The model under review builds one solid part; all positions refer to its coordinate system, in mm. A direction names the side the tool comes from. Give positions to 0.01 mm unless a question says otherwise; leave off trailing zeros. Order: outer loops, then holes, each group sorted by start corner. A loop starts at its lowest first (then second) coordinate and runs counter-clockwise, first axis right, second up.
```python
from build123d import *

# Parameters (mm, degrees)
F0_R        = 18.7
F0_R_2      = 15.45
F1_DEPTH    = 20
F0_R_3      = 21
F2_DEPTH    = 5
F3_DEPTH    = 20
F4_S5_R     = 18.7
F4_T6_DEPTH = 31
F5_SIZE     = 3


# Not quite as in the source:
# - a fillet or chamfer that OpenCascade refuses, or shapes differently, is made with other operations: its cross-section is extruded or revolved along the edge and cut away or added


with BuildPart() as f1:
    # F0 (on Top) → F1 (new body)
    with BuildSketch(Plane.XY):
        Circle(F0_R)
        Circle(F0_R_2, mode=Mode.SUBTRACT)
    extrude(amount=F1_DEPTH)

    # F0 (on Top) → F2 (join)
    with BuildSketch(Plane.XY):
        Circle(F0_R_3)
        Circle(F0_R, mode=Mode.SUBTRACT)
    extrude(amount=F2_DEPTH)

    # F0 (on Top) → F3 (join)
    with BuildSketch(Plane.XY):
        Circle(F0_R_3)
        Circle(F0_R, mode=Mode.SUBTRACT)
    extrude(amount=-F3_DEPTH)

    # F4: chamfer of 2.5 on 1 edges, made by hand


with BuildPart() as f4_tool2:
    # F4_s3 → F4_t4 (revolve)
    with BuildSketch(Plane.XZ):
        Polygon((18.5, 5), (21, 2.5), (21, 5), align=None)
    revolve(axis=Axis((0, 0, 5), (0, 0, 1)))

    # F4_s5 → F4_t6 (cut, symmetric)
    with BuildSketch(Plane.XY.offset(3.8)):
        Circle(F4_S5_R)
    extrude(amount=F4_T6_DEPTH, both=True, mode=Mode.SUBTRACT)


with BuildPart() as f1_1:
    add(f1.part)

    # F4_t1: cut F4_tool2
    add(f4_tool2.part, mode=Mode.SUBTRACT)

    # F5
    f5_edges = [f1_1.edges().sort_by_distance(p)[0] for p in [
        (-15.45, 0, 0),
    ]]
    chamfer(f5_edges, length=F5_SIZE)


solid = f1_1.part
```
Item 1: Draft analysis for pull direction X (two halves, no side actions). For faces 1 (the cylindrical face through (20.03, 6.31, -8.59)), 2 (the conical face through (-3.381, -15.225, 2.854)), 3 (the flat face through (-7, 14, 20)), state which applies: released by +X, released by -X, zero draft, split by the parting line, or undercut.
Values found:
face 1: split by the parting line
face 2: undercut
face 3: zero draft
Item 2: For line 1 (X direction, y = -0.5, z = 14); line 2 (X direction, y = -17, z = -5); line 3 (Y direction, x = 0, z = -9), list the stretches that pass through material, from the lowest coordinate up.
Values found:
line 1: x = -18.69 to -15.44, 15.44 to 18.69
line 2: x = -12.33 to -7.79, 7.79 to 12.33
line 3: y = -21 to -18.7, 18.7 to 21
Item 3: Take a section at D-D (z = 9.5). Give the boundary of the cut face in (x, y), and give its area (3 significant figures).
Values found:
outline: circle Ø37.4 at (0, 0); hole circle Ø30.9 at (0, 0)
area: 349 mm2
Item 4: Take a section at A-A (x = 0). Give the boundary of the cut face in (y, z).
Values found:
outline: (-21, -20) - (-18.7, -20) - (-18.7, 0) - (-18.45, 0) - (-15.45, 3) - (-15.45, 20) - (-18.7, 20) - (-18.7, 4.8) - (-21, 2.5) - close; (15.45, 3) - (18.45, 0) - (18.7, 0) - (18.7, -20) - (21, -20) - (21, 2.5) - (18.7, 4.8) - (18.7, 20) - (15.45, 20) - close
Item 5: Clearance check with flat-ended pins moving along their axes: pin 1 Ø6 at (x, z) = (16.5, -13) entering from +Y; pin 2 Ø1.5 at (y, z) = (-9.5, 10.5) entering from -X; pin 3 Ø3 at (x, y) = (15.5, -12) entering from +Z; pin 4 Ø5 at (x, z) = (-2.5, 12.5) entering from -Y. State where each tip first meets the part, or that it passes through.
Values found:
pin 1: stops at y = 16.09
pin 2: stops at x = -16.53
pin 3: stops at z = 20
pin 4: stops at y = -18.7
Item 6: For faces 4 (the conical face through (-14.954, -11.466, 4.656)), 5 (the cylindrical face through (-4.054, -18.255, -9.86)), list the 3-axis set-ups (+Z, -Z, +X, -X, +Y, -Y) from which the entire face can be reached by the end or side of a thin tool; tool diameter is ignored.
Values found:
face 4: +Z
face 5: -Z
Item 7: Take a section at C-C (z = -9). Give the boundary of the cut face in (x, y), and give its area (3 significant figures).
Values found:
outline: circle Ø42 at (0, 0); hole circle Ø37.4 at (0, 0)
area: 287 mm2
